Drawing for the job (mm, zero at the part's lowest x, y, z). Coordinates: 2 decimals unless noted, no trailing zeros. Loops run counter-clockwise (first coordinate to the right, second up) from the corner with the lowest first, then second, coordinate; pieces in that order, holes last. Notation, with made-up numbers: (-18.75, 22) -> (-12.75, 22) arc R8 ccw to (-12.75, 34) -> close; hole circle Ø1 at (-13.5, -39.75). An arc over 180 degrees is marked (long way). Write each question's results on one line, items separated by ' | '.
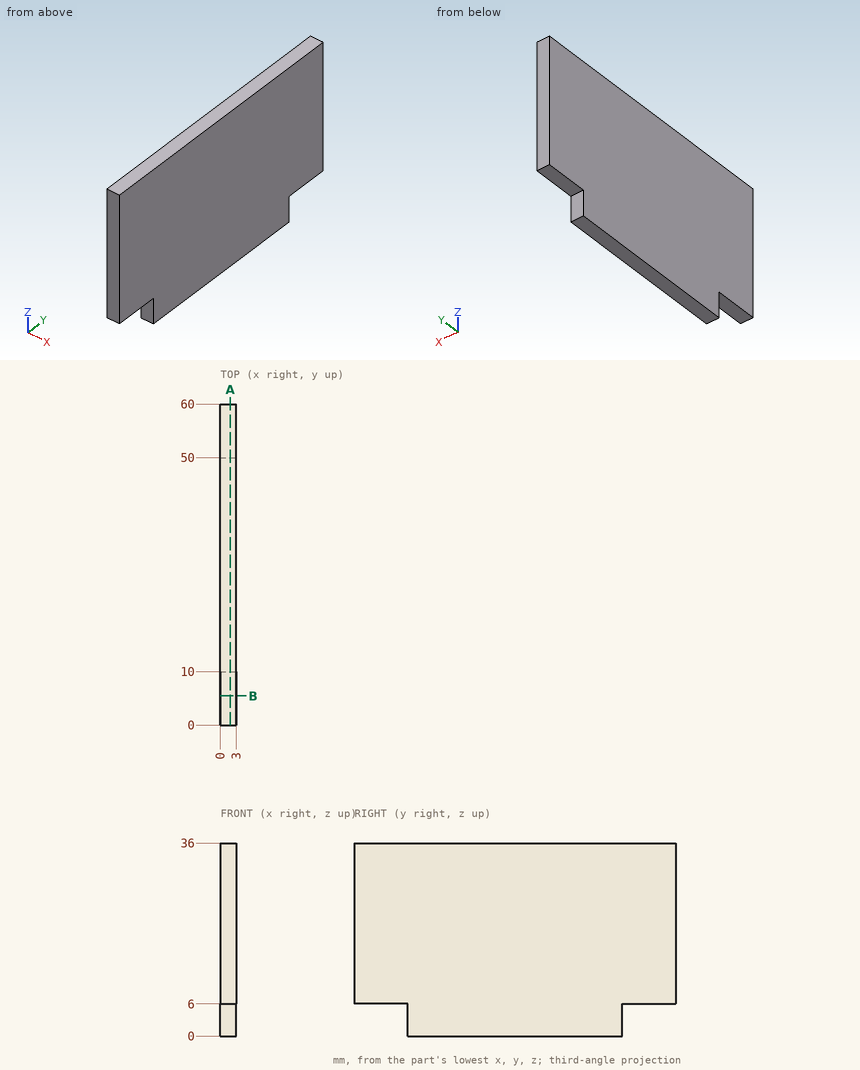
1) Slice it at B-B (y = 5.5). Write the cut outline in (x, z).
Outcome:
outline: (0, 6) -> (3, 6) -> (3, 36) -> (0, 36) -> close
2) Pin check, flat tips, straight feed: pin 1 (0.9 mm diameter, centred on x = 1.5, z = 3.5, fed in from -Y); pin 2 (1.5 mm diameter, centred on x = 1, y = 3, fed in from -Z). Stop position of each tip, or through.
Outcome:
pin 1: stops at y = 10 | pin 2: stops at z = 6
3) Slice it at A-A (x = 1.85). Write the cut outline in (y, z), then the cut area to 3 significant figures.
Outcome:
outline: (0, 6) -> (10, 6) -> (10, 0) -> (50, 0) -> (50, 6) -> (60, 6) -> (60, 36) -> (0, 36) -> close | area: 2,040 mm^2
4) Drill centre lines: L1, parallel to Z at x = 0.3, y = 8; L2, parallel to Y at x = 0.5, z = 1. Where is each one in solid material? Low to high. Write a range as from..to.
Outcome:
L1: z = 6..36 | L2: y = 10..50
